Source: CAD feature listing. Evaluate the final solid. Frame: model axes, mm. A direction names the side the tool comes from. Give positions to 0.01 mm unless a question says otherwise; leave off trailing zeros. Loops run counter-clockwise (first coordinate to the right, second up) from the corner with the lowest first, then second, coordinate; pieces in that order, holes last.
from build123d import *

# Parameters (mm, degrees)
F1_R     = 10.2
F2_DEPTH = 20
F3_R     = 17.5
F4_DEPTH = 1
F6_D     = 12.9
F7_SIZE2 = 0.2
F7_SIZE  = 0.2
F8_SIZE2 = 1.8660254038
F8_SIZE  = 0.5


with BuildPart() as f2:
    # F1 (on Top) → F2 (new body)
    with BuildSketch(Plane.XY):
        Circle(F1_R)
    extrude(amount=F2_DEPTH)

    # F3 (on face) → F4 (join)
    with BuildSketch(Plane(origin=(0, 0, 0), x_dir=(1, 0, 0), z_dir=(0, 0, -1))):
        Circle(F3_R)
    extrude(amount=F4_DEPTH)

    # F6 (through all)
    with Locations(Plane(origin=(0, 0, -1), x_dir=(1, 0, 0), z_dir=(0, 0, -1))):
        with Locations((0, 0)):
            Hole(F6_D / 2)

    # F7
    f7_edges = [f2.edges().sort_by_distance(p)[0] for p in [
        (-17.5, 0, -1),
    ]]
    chamfer(f7_edges, length=F7_SIZE, length2=F7_SIZE2)

    # F8
    f8_edges = [f2.edges().sort_by_distance(p)[0] for p in [
        (-10.2, 0, 20),
    ]]
    f8_side = f2.faces().sort_by_distance((-9.9115, 0, 20))[0]
    chamfer(f8_edges, length=F8_SIZE, length2=F8_SIZE2, reference=f8_side)


solid = f2.part
1) Pull-direction query (Y, two-part tool) for faces 1 (the flat face through (6.3, -2, 20)), 2 (the cylindrical face through (1.398, 6.297, 9.647)), 3 (the cylindrical face through (4.707, -9.049, 8.94)); classes: released by +Y, released by -Y, zero draft, split by the parting line, or undercut.
Checks:
face 1: zero draft
face 2: undercut
face 3: split by the parting line
2) Reachability of faces 4 (the flat face through (8, 8, 0)), 5 (the flat face through (7, 0, -1)) from +Z, -Z, +X, -X, +Y, -Y: full face, straight path, thin tool, end or side. Return the list, or none.
Checks:
face 4: +Z
face 5: -Z, +X, -X, +Y, -Y
3) Ray query, probe 1 along Y at (x, z) = (0, 3.5); probe 2 along X at (y, z) = (5, 8.25); probe 3 along X at (y, z) = (4, 6.5). Return the intervals inside material, ascending.
Checks:
probe 1: y = -10.2 to -6.45, 6.45 to 10.2
probe 2: x = -8.89 to -4.07, 4.07 to 8.89
probe 3: x = -9.38 to -5.06, 5.06 to 9.38
4) Contact query for flat-ended pins moving along their axis: P1, Ø2, axis at y = 6.5, z = 7, coming from the -X side; P2, Ø17, axis at x = 0, y = 0, coming from the +Z side; P3, Ø3, axis at x = 4.5, z = 2, coming from the -Y side; P4, Ø1, axis at x = -3, z = 8, coming from the -Y side. Output: stop coordinate, or through.
Checks:
P1: stops at x = -8.59
P2: stops at z = 20
P3: stops at y = -9.75
P4: stops at y = -9.89
5) Cut plane C-C (z = 16). Return loops of the section in (x, y).
Checks:
outline: circle Ø20.4 at (0, 0); hole circle Ø12.9 at (0, 0)
6) Cut plane A-A (y = 0). Return loops of the section in (x, z).
Checks:
outline: (-17.5, -0.8) - (-17.3, -1) - (-6.45, -1) - (-6.45, 20) - (-9.7, 20) - (-10.2, 18.13) - (-10.2, 0) - (-17.5, 0) - close; (6.45, -1) - (17.3, -1) - (17.5, -0.8) - (17.5, 0) - (10.2, 0) - (10.2, 18.13) - (9.7, 20) - (6.45, 20) - close
